```python
from build123d import *

# Parameters (mm, degrees)
SKETCH1_R           = 1.5
SKETCH1_R_2         = 2
SKETCH1_W           = 20
SKETCH1_H           = 40
BOSS_EXTRUDE1_DEPTH = 5


with BuildPart() as part:
    # Sketch1 → Boss-Extrude1 (new body)
    with BuildSketch(Plane(origin=(0, 0, 0), x_dir=(1, 0, 0), z_dir=(0, 1, 0))):
        Polygon((5, 0), (19, 0), (19, 5), (24, 5), (24, 62.5), (19, 62.5), (19, 67.5), (5, 67.5), (5, 62.5), (0, 62.5), (0, 5), (5, 5), align=None)
        with Locations(Location((12, 65, 0), (0, 0, 270))):
            Circle(SKETCH1_R, mode=Mode.SUBTRACT)
        with Locations(Location((12, 2.5, 0), (0, 0, 90))):
            Circle(SKETCH1_R, mode=Mode.SUBTRACT)
        with Locations(Location((16.75, 58, 0), (0, 0, 270))):
            Circle(SKETCH1_R_2, mode=Mode.SUBTRACT)
        with Locations(Location((7.25, 58, 0), (0, 0, 90))):
            Circle(SKETCH1_R_2, mode=Mode.SUBTRACT)
        with Locations(Location((16.75, 9.5, 0), (0, 0, 90))):
            Circle(SKETCH1_R_2, mode=Mode.SUBTRACT)
        with Locations(Location((7.25, 9.5, 0), (0, 0, 270))):
            Circle(SKETCH1_R_2, mode=Mode.SUBTRACT)
        with Locations((12, 33.75)):
            Rectangle(SKETCH1_W, SKETCH1_H, mode=Mode.SUBTRACT)
    extrude(amount=BOSS_EXTRUDE1_DEPTH)


solid = part.part
```
CAD build for the part. Positions are in the model's coordinates, mm. A direction names the side the tool comes from. Round coordinates to 2 decimals unless told otherwise and drop trailing zeros. Write each loop counter-clockwise with the first axis right and the second up, starting at its lowest first coordinate (ties: lowest second). Pieces come first, ordered by that corner, then holes.
Item 1: Band-saw the part on B-B on z = -14.5. Write the cut outline in (x, y), then the cut area to 3 significant figures.
Filled in:
outline: (0, 0) - (2, 0) - (2, 5) - (0, 5) - close; (22, 0) - (24, 0) - (24, 5) - (22, 5) - close
area: 20.0 mm2
Item 2: Mould opens along X. For faces 1 (the cylindrical face through (6.649, 2.465, -59.908)), 2 (the cylindrical face through (12.45, 2.46, -63.57)), 3 (the flat face through (24, 2, -33)), 4 (the flat face through (0, 2, -34)) say: released by +X, released by -X, zero draft, split by the parting line, or undercut.
Filled in:
face 1: undercut
face 2: undercut
face 3: released by +X
face 4: released by -X
Item 3: Band-saw the part on C-C on y = 1.5. Write the cut outline in (x, z).
Filled in:
outline: (0, -62.5) - (5, -62.5) - (5, -67.5) - (19, -67.5) - (19, -62.5) - (24, -62.5) - (24, -5) - (19, -5) - (19, 0) - (5, 0) - (5, -5) - (0, -5) - close; hole (2, -53.75) - (22, -53.75) - (22, -13.75) - (2, -13.75) - close; hole circle Ø4 at (7.25, -58); hole circle Ø4 at (7.25, -9.5); hole circle Ø3 at (12, -65); hole circle Ø3 at (12, -2.5); hole circle Ø4 at (16.75, -58); hole circle Ø4 at (16.75, -9.5)
Item 4: Tool access for faces 5 (the flat face through (21, 2, -5)), 6 (the flat face through (12, 2, -53.75)), 7 (the flat face through (2, 2, -5)), 8 (the flat face through (22, 2, -62.5)): list every direction of +Z, -Z, +X, -X, +Y, -Y with a clear straight run to the whole face (end or side of a thin tool).
Filled in:
face 5: +Z, +X, +Y, -Y
face 6: +Y, -Y
face 7: +Z, -X, +Y, -Y
face 8: -Z, +X, +Y, -Y
Item 5: Drop flat-ended pins along their axis: pin 1 Ø1.5 at (x, y) = (3, 2.5) entering from -Z; pin 2 Ø3 at (x, z) = (16.75, -58) entering from +Y; pin 3 Ø2.5 at (x, y) = (2, 2.5) entering from +Z; pin 4 Ø1.5 at (y, z) = (3, -66) entering from -X. Give the stop position or say it passes through.
Filled in:
pin 1: stops at z = -62.5
pin 2: passes through
pin 3: stops at z = -5
pin 4: stops at x = 5
Item 6: Drill centre lines: L1, parallel to X at y = 2.8, z = -58; L2, parallel to X at y = 2.55, z = -36; L3, parallel to Z at x = 18, y = 0.65. Where is each one in solid material? Low to high.
Filled in:
L1: x = 0 to 5.25, 9.25 to 14.75, 18.75 to 24
L2: x = 0 to 2, 22 to 24
L3: z = -67.5 to -59.56, -56.44 to -53.75, -13.75 to -11.06, -7.94 to 0
Item 7: Band-saw the part on A-A on x = 4.25. Write the cut outline in (y, z).
Filled in:
outline: (0, -62.5) - (5, -62.5) - (5, -53.75) - (0, -53.75) - close; (0, -13.75) - (5, -13.75) - (5, -5) - (0, -5) - close
Item 8: Band-saw the part on D-D on x = 12. Write the cut outline in (y, z).
Filled in:
outline: (0, -67.5) - (5, -67.5) - (5, -66.5) - (0, -66.5) - close; (0, -63.5) - (5, -63.5) - (5, -53.75) - (0, -53.75) - close; (0, -13.75) - (5, -13.75) - (5, -4) - (0, -4) - close; (0, -1) - (5, -1) - (5, 0) - (0, 0) - close
